Verification items for the finished model (mm, model axes). Round coordinates to 2 decimals unless told otherwise and drop trailing zeros. Write each loop counter-clockwise with the first axis right and the second up, starting at its lowest first coordinate (ties: lowest second). Pieces come first, ordered by that corner, then holes. Notation, with made-up numbers: M -23,-31 L 0,-31 A14 ccw 0,-19 Z; hole C 19.5,-12 d5. An arc over 180 degrees is marked long. Use a Markdown table: item, result. Add a question column.
from build123d import *

# Parameters (mm, degrees)
F0_R     = 17.4625
F1_DEPTH = 4.7625
F2_D     = 10.71626
F3_R     = 6.35
F5_D     = 9.525


with BuildPart() as f1:
    # F0 (on Top) → F1 (new body)
    with BuildSketch(Plane.XY):
        with BuildLine():
            ThreePointArc((-25.4, 42.161447), (-26.591422, 37.216961), (-29.627334, 33.136438))
            ThreePointArc((-29.627334, 33.136438), (0, -44.45), (29.627334, 33.136438))
            ThreePointArc((29.627334, 33.136438), (26.591422, 37.216961), (25.4, 42.161447))
            Line((25.4, 42.161447), (12.7, 406.4))
            Line((12.7, 406.4), (-12.7, 406.4))
            Line((-12.7, 406.4), (-25.4, 42.161447))
        make_face()
        Circle(F0_R, mode=Mode.SUBTRACT)
    extrude(amount=-F1_DEPTH)

    # F2 (through all)
    with Locations(Plane.XY):
        with Locations((0, 31.75), (31.75, 0), (0, -31.75), (-31.75, 0)):
            Hole(F2_D / 2)

    # F3
    f3_edges = [f1.edges().sort_by_distance(p)[0] for p in [
        (-12.7, 406.4, -2.38125),
        (12.7, 406.4, -2.38125),
    ]]
    fillet(f3_edges, radius=F3_R)

    # F5 (through all)
    with Locations(Plane.XY):
        with Locations((-26.940768, 26.940768), (26.940768, 26.940768), (26.940768, -26.940768), (-26.940768, -26.940768)):
            Hole(F5_D / 2)


solid = f1.part
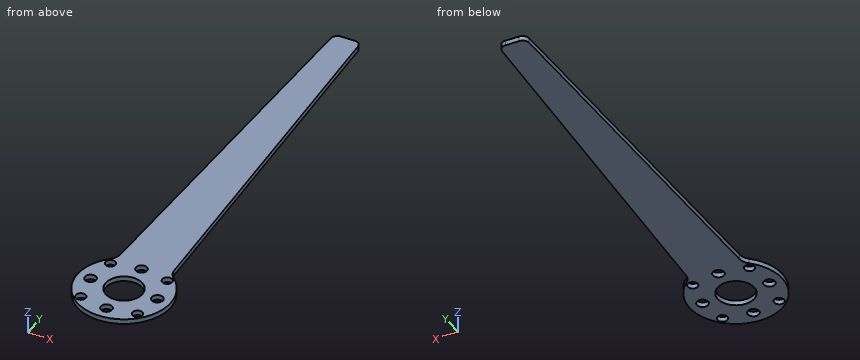
1. Cross-section at C-C on z = -2.35. Count the separate pieces of the cut face and the enclosed holes in it, plus the area to 3 significant figures.
2. Cross-section at A-A on y = 0. Enter the section's corners in (x, z).
3. Cross-section at B-B on x = 0. Enter the section's corners in (y, z).
4. Cross-section at D-D on y = 199.5. Enter the section's corners in (x, z).
5. Depth check by flat-ended pin: pin 1 Ø5.5 at (x, y) = (-26.94, 26.94) entering from +Z; pin 2 Ø1.5 at (x, z) = (33.5, -1) entering from +Y. Enter the tip coordinate at first touch or a pass-through.
6. Scan lines: line 1 along Y through (x, z) = (0, -3.75); line 2 along Y through (x, z) = (6.5, -1.15); line 3 along Y through (x, z) = (-31, -1.55). Record each from-to range of solid material in increasing order. Write a range as from..to.
Answer:
| question | item | result |
|---|---|---|
| 1 | separate pieces | 1 |
| 1 | enclosed holes | 9 |
| 1 | area | 18,500 mm^2 |
| 2 | outline | M -44.45,-4.76 L -37.11,-4.76 L -37.11,0 L -44.45,0 Z; M -26.39,-4.76 L -17.46,-4.76 L -17.46,0 L -26.39,0 Z; M 17.46,-4.76 L 26.39,-4.76 L 26.39,0 L 17.46,0 Z; M 37.11,-4.76 L 44.45,-4.76 L 44.45,0 L 37.11,0 Z |
| 3 | outline | M -44.45,-4.76 L -37.11,-4.76 L -37.11,0 L -44.45,0 Z; M -26.39,-4.76 L -17.46,-4.76 L -17.46,0 L -26.39,0 Z; M 17.46,-4.76 L 26.39,-4.76 L 26.39,0 L 17.46,0 Z; M 37.11,-4.76 L 406.4,-4.76 L 406.4,0 L 37.11,0 Z |
| 4 | outline | M -19.91,-4.76 L 19.91,-4.76 L 19.91,0 L -19.91,0 Z |
| 5 | pin 1 | passes through |
| 5 | pin 2 | stops at y = 30.05 |
| 6 | line 1 | y = -44.45..-37.11, -26.39..-17.46, 17.46..26.39, 37.11..406.4 |
| 6 | line 2 | y = -43.97..-16.21, 16.21..406.4 |
| 6 | line 3 | y = -31.86..-29.43, -24.45..-5.31, 5.31..24.45, 29.43..31.86 |
